The listing builds one solid part. Answer for the finished solid, in the listing's coordinates (mm). A direction names the side the tool comes from. Coordinates: 2 decimals unless noted, no trailing zeros. Loops run counter-clockwise (first coordinate to the right, second up) from the corner with the lowest first, then second, coordinate; pieces in that order, holes last. Notation, with made-up numbers: (-32.75, -10) - (25.25, -10) arc R6 cw to (25.25, -2) - close; hole circle Ø7 at (29.5, 71.25). An arc over 180 degrees is marked (long way). Return JSON: item names as keys, results as strings. Group by question number.
1. Find the intervals of material crossed by line 1 along X through (y, z) = (-9, 13.5); line 2 along Y through (x, z) = (13, 1.5); line 3 along Y through (x, z) = (-6, 14.75), in increasing order.
2. Each of these flat-tipped pins is pushed along its axis until it touches: P1, Ø2, axis at y = 10.5, z = 13.5, coming from the +X side; P2, Ø4.5, axis at x = -6, y = 10.39, coming from the +Z side; P3, Ø2, axis at x = 16, z = 4, coming from the +Y side; P4, Ø8, axis at x = -11.5, z = 12.5, coming from the +Y side. Where does it stop, or does it pass through?
3. Which of the six approach directions +Z, -Z, +X, -X, +Y, -Y give full straight-line access (tool end or side, diameter ignored) to faces 1 (the face through (-10, 3.2, 2.5)), 2 (the face through (0, -12, 0)), 3 (the face through (-4.784, 11.507, 15.944))?
4. Section A-A (x = -20.65) is taken. Write down the section's boundary in (y, z).
5. Section B-B (x = 0) is taken. Write down the section's boundary in (y, z).
6. Section D-D (z = 3.5) is taken. Write down the section's boundary in (x, y) (3 decimals).
7. Section C-C (z = 14.25) is taken. Write down the section's boundary in (x, y).
8. The mould has two halves that part along X. Classify faces 4 (the face through (0, 0, 20)), 5 (the face through (-7.554, -19.032, 3.451)), 6 (the face through (-5.961, -26.846, 3.451)), 7 (the face through (1.172, 8.923, 5.74)): pulls with the +X half, pulls with the -X half, needs draft (parallel to the pull), parting line crosses it, or undercut.
```python
from build123d import *

# Parameters (mm, degrees)
SKETCH1_R             = 27.5
SKETCH1_R_2           = 3
BOSS_EXTRUDE1_DEPTH   = 7
SKETCH2_R             = 10.5
CUT_EXTRUDE1_DEPTH    = 5
SKETCH4_R             = 17.5
BOSS_EXTRUDE2_DEPTH   = 13
SKETCH6_R             = 9
CUT_EXTRUDE3_DEPTH    = 1.5
M4_TAPPED_HOLE1_D     = 3.3
M4_TAPPED_HOLE1_DEPTH = 8
M4_TAPPED_HOLE1_TIP   = 0.991420021


with BuildPart() as part:
    # Sketch1 → Boss-Extrude1 (new body)
    with BuildSketch(Plane.XY):
        Circle(SKETCH1_R)
        with Locations((20.65, 0)):
            Circle(SKETCH1_R_2, mode=Mode.SUBTRACT)
        with Locations((10.325, -17.883424588)):
            Circle(SKETCH1_R_2, mode=Mode.SUBTRACT)
        with Locations((-10.325, -17.883424588)):
            Circle(SKETCH1_R_2, mode=Mode.SUBTRACT)
        with Locations((-20.65, 0)):
            Circle(SKETCH1_R_2, mode=Mode.SUBTRACT)
        with Locations((-10.325, 17.883424588)):
            Circle(SKETCH1_R_2, mode=Mode.SUBTRACT)
        with Locations((10.325, 17.883424588)):
            Circle(SKETCH1_R_2, mode=Mode.SUBTRACT)
    extrude(amount=BOSS_EXTRUDE1_DEPTH)

    # Sketch2 → Cut-Extrude1 (cut)
    with BuildSketch(Plane(origin=(0, 0, 0), x_dir=(-1, 0, 0), z_dir=(0, 0, -1))):
        Circle(SKETCH2_R)
    extrude(amount=-CUT_EXTRUDE1_DEPTH, mode=Mode.SUBTRACT)

    # Sketch4 → Boss-Extrude2 (add)
    with BuildSketch(Plane.XY.offset(7)):
        with Locations(Location((0, 0, 0), (0, 0, 180))):
            Circle(SKETCH4_R)
    extrude(amount=BOSS_EXTRUDE2_DEPTH)

    # Sketch6 → Cut-Extrude3 (cut)
    with BuildSketch(Plane(origin=(0, 0, 5), x_dir=(-1, 0, 0), z_dir=(0, 0, -1))):
        Circle(SKETCH6_R)
    extrude(amount=-CUT_EXTRUDE3_DEPTH, mode=Mode.SUBTRACT)

    # M4 Tapped Hole1
    with Locations(Plane(origin=(-6, 10.392304845, 20), x_dir=(1, 0, 0), z_dir=(0, 0, 1))):
        with Locations((0, 0), (12, 0), (18, -10.392304845), (12, -20.78460969), (0, -20.78460969), (-6, -10.392304845)):
            Hole(M4_TAPPED_HOLE1_D / 2, depth=M4_TAPPED_HOLE1_DEPTH)
            with Locations((0, 0, -(M4_TAPPED_HOLE1_DEPTH + M4_TAPPED_HOLE1_TIP / 2))):  # 118° drill point
                Cone(0, M4_TAPPED_HOLE1_D / 2, M4_TAPPED_HOLE1_TIP, mode=Mode.SUBTRACT)


solid = part.part
```
The answers:
{
 "1": {"line 1": "x = -15.01 to -6.89, -5.11 to 5.11, 6.89 to 15.01", "line 2": "y = -24.23 to -19.24, -16.53 to 16.53, 19.24 to 24.23", "line 3": "y = -16.44 to -12.04, -8.74 to 8.74, 12.04 to 16.44"},
 "2": {"P1": "stops at x = 14.7", "P2": "stops at z = 20", "P3": "stops at y = 23.05", "P4": "stops at y = 15.81"},
 "3": {"face 1": "-Z", "face 2": "-Z, +X, -X, +Y, -Y", "face 3": "+Z"},
 "4": {"outline": "(-18.16, 0) - (-3, 0) - (-3, 7) - (-18.16, 7) - close; (3, 0) - (18.16, 0) - (18.16, 7) - (3, 7) - close"},
 "5": {"outline": "(-27.5, 0) - (-10.5, 0) - (-10.5, 5) - (-9, 5) - (-9, 6.5) - (9, 6.5) - (9, 5) - (10.5, 5) - (10.5, 0) - (27.5, 0) - (27.5, 7) - (17.5, 7) - (17.5, 20) - (-17.5, 20) - (-17.5, 7) - (-27.5, 7) - close"},
 "6": {"outline": "circle Ø55 at (0, 0); hole circle Ø6 at (-20.65, 0); hole circle Ø6 at (-10.325, -17.883); hole circle Ø6 at (-10.325, 17.883); hole circle Ø21 at (0, 0); hole circle Ø6 at (10.325, -17.883); hole circle Ø6 at (10.325, 17.883); hole circle Ø6 at (20.65, 0)"},
 "7": {"outline": "circle Ø35 at (0, 0); hole circle Ø3.3 at (-12, 0); hole circle Ø3.3 at (-6, -10.39); hole circle Ø3.3 at (-6, 10.39); hole circle Ø3.3 at (6, -10.39); hole circle Ø3.3 at (6, 10.39); hole circle Ø3.3 at (12, 0)"},
 "8": {"face 4": "needs draft", "face 5": "undercut", "face 6": "parting line crosses it", "face 7": "undercut"}
}
